Build history of the part. All positions in model axes, mm. Face numbers are marked on the shaded views. A direction names the side the tool comes from. Round coordinates to 2 decimals unless told otherwise and drop trailing zeros. Write each loop counter-clockwise with the first axis right and the second up, starting at its lowest first coordinate (ties: lowest second). Pieces come first, ordered by that corner, then holes.
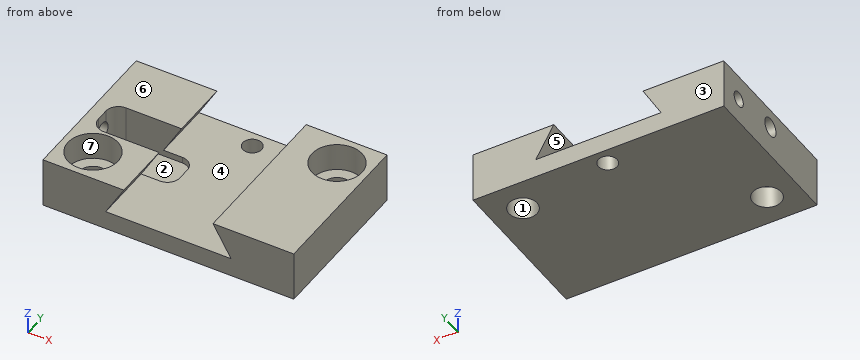
Autodesk Inventor part; units mm, degrees
ref_plane "YZ Plane" through (0, 0, 0) normal (1, 0, 0) x (0, 1, 0)
ref_plane "XZ Plane" through (0, 0, 0) normal (0, 1, 0) x (-1, 0, 0)
ref_plane "XY Plane" through (0, 0, 0) normal (0, 0, 1) x (1, 0, 0)
sketch "Skizze1" plane through (0, 0, 0) normal (0, 0, 1) x (1, 0, 0)
  line L0 (-20, 12.5) -> (20, 12.5)
  line L1 (20, 12.5) -> (20, -12.5)
  line L2 (20, -12.5) -> (-20, -12.5)
  line L3 (-20, -12.5) -> (-20, 12.5)
  line L4 (-28, 0) -> (28, 0)
  line L5 (0, -17.5) -> (0, 17.5)
  point P0 (0, 0)
  dimension "d0" = 40
  dimension "d1" = 25
extrude "Extrusion1" add sketch "Skizze1" along normal blind 8
sketch "Skizze2" plane through (0, 0, 8) normal (0, 0, 1) x (1, 0, 0)
  line L0 (-28, 0) -> (28, 0)
  line L1 (0, -17.5) -> (0, 17.5)
  line L2 (-15, 7.5) -> (15, 7.5)
  line L3 (15, 7.5) -> (15, -7.5)
  line L4 (15, -7.5) -> (-15, -7.5)
  line L5 (-15, -7.5) -> (-15, 7.5)
  point P0 (0, 0)
  dimension "d4" = 15
  dimension "d5" = 30
hole "Bohrung1" at (-15, -7.5, 8) at (15, 7.5, 8) direction (0, 0, -1) diameter 4.5 end through all counterbore diameter 8 counterbore depth 4.4
sketch "Skizze5" plane through (-20, -12.5, 0) normal (0, -1, 0) x (1, 0, 0)
  line L0 (40, 8) -> (0, 8)
  line L1 (-8, 0) -> (48, 0)
  line L2 (20, -1.6) -> (20, 9.6)
  line L3 (12.8868, 8) -> (27.1132, 8)
  line L4 (27.1132, 8) -> (30, 3)
  line L5 (30, 3) -> (10, 3)
  line L6 (10, 3) -> (12.8868, 8)
  point P0 (20, 0)
  dimension "d37" = 5
  dimension "d38" = 60
  dimension "d39" = 20
extrude "Extrusion2" cut sketch "Skizze5" against normal through all
sketch "Skizze6" plane through (0, 0, 0) normal (0, 0, -1) x (-1, 0, 0)
  line L0 (28, 0) -> (-28, 0)
  line L1 (0, -17.5) -> (0, 17.5)
  point P0 (0, 0)
  point P1 (0, 10)
  dimension "d42" = 10
hole "Bohrung5" at (0, 10, 0) direction (0, 0, 1) diameter 3 end through all
sketch "Skizze7" plane through (0, 0, 8) normal (0, 0, 1) x (1, 0, 0)
  line L0 (-20, -12.5) -> (-20, 12.5)
  line L1 (-28, 0) -> (28, 0)
  line L2 (0, -17.5) -> (0, 17.5)
  line L3 (-16, 3) -> (-7, 3)
  line L4 (-5, 1) -> (-5, -1)
  line L5 (-7, -3) -> (-16, -3)
  line L6 (-18, -1) -> (-18, 1)
  arc A0 (-16, 3) -> (-18, 1) centre (-16, 1) ccw
  arc A1 (-18, -1) -> (-16, -3) centre (-16, -1) ccw
  arc A2 (-7, -3) -> (-5, -1) centre (-7, -1) ccw
  arc A3 (-5, 1) -> (-7, 3) centre (-7, 1) ccw
  point P0 (0, 0)
  dimension "d53" = 2
  dimension "d54" = 15
  dimension "d55" = 13
  dimension "d56" = 2
  dimension "d57" = 6
extrude "Extrusion3" cut sketch "Skizze7" against normal blind 6
sketch "Skizze8" plane through (-20, -12.5, 0) normal (-1, 0, 0) x (0, 0, 1)
  line L0 (8, 0) -> (8, 25)
  line L1 (8, 15.5) -> (3, 15.5)
  line L2 (8, 15.5) -> (2, 15.5)
  line L3 (3, 15.5) -> (2, 15.5)
  line L4 (3.6, 1) -> (3.6, 9)
  line L5 (3, 9.5) -> (2, 9.5)
  line L6 (8, 9.5) -> (2, 9.5)
  line L7 (3, 9.5) -> (8, 9.5)
  line L8 (0, -5) -> (0, 30)
  line L9 (-1.6, 12.5) -> (9.6, 12.5)
  point P0 (0, 12.5)
  point P1 (5, 12.5)
  dimension "d60" = 3
hole "Bohrung6" at (-20, 0, 5) direction (1, 0, 0) diameter 3 depth 3 tip angle 118
hole "Bohrung7" at (-20, 8.5, 4) direction (1, 0, 0) diameter 2.459 depth 8 tip angle 118
properties part number "13_1087_032"
1) Slice it at D-D (y = 0.5). Write the cut outline in (x, z).
Results:
outline: (-20, 0) - (20, 0) - (20, 8) - (7.11, 8) - (10, 3) - (-5, 3) - (-5, 2) - (-18, 2) - (-18, 3.59) - (-20, 3.59) - close; (-20, 6.41) - (-18, 6.41) - (-18, 8) - (-20, 8) - close
2) Pin check, flat tips, straight feed: pin 1 Ø1.5 at (x, y) = (8, 5.5) entering from -Z; pin 2 Ø6 at (x, y) = (1.5, -3.5) entering from +Z. Stop position of each tip, or through.
Results:
pin 1: stops at z = 0
pin 2: stops at z = 3
3) Mould opens along Y. For the marked faces 1, 2, 3 and 4 say: released by +Y, released by -Y, zero draft, split by the parting line, or undercut.
Results:
face 1: undercut
face 2: undercut
face 3: released by +Y
face 4: zero draft
4) Wall check: L1, parallel to Z at x = -19.25, y = 0; L2, parallel to Y at x = 15, z = 2.7; L3, parallel to X at y = -11, z = 3.75. Give the ranges that are in metal, low to high.
Results:
L1: z = 0 to 3.5, 6.5 to 8
L2: y = -12.5 to 5.25, 9.75 to 12.5
L3: x = -20 to -16.94, -13.06 to -9.57, 9.57 to 20
5) Which spindle directions (+Z, -Z, +X, -X, +Y, -Y) get a long thin tool onto all of the face, cutting with end or side? Do the marked faces 5, 6 and 7. Say none if no direction does.
Results:
face 5: +Y, -Y
face 6: +Z, +X, -X, +Y, -Y
face 7: +Z
6) Slice it at C-C (x = 15). Write the cut outline in (y, z).
Results:
outline: (-12.5, 0) - (5.25, 0) - (5.25, 3.6) - (3.5, 3.6) - (3.5, 8) - (-12.5, 8) - close; (9.75, 0) - (12.5, 0) - (12.5, 8) - (11.5, 8) - (11.5, 3.6) - (9.75, 3.6) - close
7) Slice it at A-A (x = -15). Write the cut outline in (y, z), plus the area to 3 significant figures.
Results:
outline: (-12.5, 0) - (-9.75, 0) - (-9.75, 3.6) - (-11.5, 3.6) - (-11.5, 8) - (-12.5, 8) - close; (-5.25, 0) - (12.5, 0) - (12.5, 8) - (3, 8) - (3, 2) - (-3, 2) - (-3, 8) - (-3.5, 8) - (-3.5, 3.6) - (-5.25, 3.6) - close; hole circle Ø2.46 at (8.5, 4)
area: 108 mm2
8) Slice it at B-B (z = 7.5). Write the cut outline in (x, y), plus the area to 3 significant figures.
Results:
outline: (-20, -12.5) - (-7.4, -12.5) - (-7.4, -3) - (-16, -3) arc R2 cw to (-18, -1) - (-18, 1) arc R2 cw to (-16, 3) - (-7.4, 3) - (-7.4, 12.5) - (-20, 12.5) - close; (7.4, -12.5) - (20, -12.5) - (20, 12.5) - (7.4, 12.5) - close; hole circle Ø8 at (-15, -7.5); hole circle Ø8 at (15, 7.5)
area: 468 mm2
